The model under review builds one solid part; all positions refer to its coordinate system, in mm. Face numbers are marked on the shaded views. A direction names the side the tool comes from. Coordinates: 2 decimals unless noted, no trailing zeros. Loops run counter-clockwise (first coordinate to the right, second up) from the corner with the lowest first, then second, coordinate; pieces in that order, holes last. Notation, with made-up numbers: (6.25, -8.75) - (20.25, -8.75) arc R19 ccw to (20.25, -4.75) - close; hole circle Ø4 at (62, 21). An arc over 180 degrees is marked (long way). Use a Markdown table: item, result. Add a question column.
1) Clearance check with flat-ended pins moving along their axes: pin 1 (6 mm diameter, centred on y = -3.5, z = -8.5, fed in from +X); pin 2 (1.5 mm diameter, centred on y = 1.5, z = 15, fed in from -X); pin 3 (3 mm diameter, centred on x = -16.5, y = 6, fed in from +Z). State where each tip first meets the part, or that it passes through.
2) To check wall thickness, follow L1, parallel to Y at x = -23.9, z = 10.35; L2, parallel to Y at x = 23, z = 9; L3, parallel to Z at x = 23.5, y = 2. State the ranges of each line that lie inside material, in increasing order. Write a range as [from, to].
3) Add section B-B, the plane y = 5.1. Give the boundary of the cut face in (x, z).
4) Add section C-C, the plane x = 8. Give the boundary of the cut face in (y, z), and give its area (3 significant figures).
5) For the marked faces 1, 2, 3 and 4, list the 3-axis set-ups (+Z, -Z, +X, -X, +Y, -Y) from which the entire face can be reached by the end or side of a thin tool; tool diameter is ignored.
6) Add section A-A, the plane x = -23.9. Give the boundary of the cut face in (y, z).
7) Add section D-D, the plane z = 10.5. Give the boundary of the cut face in (x, y).
Autodesk Inventor part; units mm, degrees
ref_plane "YZ Plane" through (0, 0, 0) normal (1, 0, 0) x (0, 1, 0)
ref_plane "XZ Plane" through (0, 0, 0) normal (0, 1, 0) x (-1, 0, 0)
ref_plane "XY Plane" through (0, 0, 0) normal (0, 0, 1) x (1, 0, 0)
sketch "草圖1" plane through (0, 0, 0) normal (0, 1, 0) x (-1, 0, 0)
  line L0 (20, -18.25) -> (-20, -18.25)
  line L1 (-20, -18.25) -> (-20, 18.25)
  line L2 (-20, 18.25) -> (20, 18.25)
  line L3 (20, 18.25) -> (20, -18.25)
  line L4 (20, -18.25) -> (-20, 18.25) construction
  line L5 (-20, -18.25) -> (20, 18.25) construction
  line L6 (26.4, 11.25) -> (-26.4, 11.25)
  line L7 (-26.4, 11.25) -> (-26.4, 8.25)
  line L8 (-26.4, 8.25) -> (26.4, 8.25)
  line L9 (26.4, 8.25) -> (26.4, 11.25)
  point P0 (0, 0)
  point P1 (0, 11.25)
  point P2 (0, 18.25)
  dimension "d0" = 40
  dimension "d1" = 36.5
  dimension "d2" = 3
  dimension "d4" = 52.8
  dimension "d5" = 26.5
extrude "擠出1" add sketch "草圖1" along normal mid plane 20
sketch "草圖2" plane through (20, -10, 11.25) normal (0, 0, 1) x (1, 0, 0)
  line L0 (-40, 0) -> (-40, 20) construction
  line L1 (0, 20) -> (-40, 20) construction
  line L2 (0, 20) -> (0, 0) construction
  line L3 (-40, 0) -> (0, 0) construction
  line L4 (-43.9, 4.9) -> (3.9, 4.9) construction
  line L5 (3.9, 4.9) -> (3.9, 15.1) construction
  line L6 (3.9, 15.1) -> (-43.9, 15.1) construction
  line L7 (-43.9, 15.1) -> (-43.9, 4.9) construction
  line L8 (-43.9, 4.9) -> (3.9, 15.1) construction
  line L9 (3.9, 4.9) -> (-43.9, 15.1) construction
  point P0 (-20, 10)
  dimension "d8" = 47.8
  dimension "d9" = 10.2
hole "孔1" at (23.9, 5.1, 11.25) at (23.9, -5.1, 11.25) at (-23.9, -5.1, 11.25) at (-23.9, 5.1, 11.25) direction (0, 0, -1) diameter 5 depth 8 tip angle 118
sketch "草圖3" plane through (20, -10, 11.25) normal (0, 0, 1) x (1, 0, 0)
  circle A0 centre (3.9, 15.1) radius 2.5 construction
  line L0 (3.9, 16.6) -> (13.7017, 16.6)
  line L1 (13.7017, 16.6) -> (13.7017, 13.6)
  line L2 (13.7017, 13.6) -> (3.9, 13.6)
  line L3 (3.9, 13.6) -> (3.9, 16.6)
  point P0 (-20, 10)
  point P1 (6.4, 15.1)
  dimension "d17" = 3
extrude "擠出2" cut sketch "草圖3" against normal blind 20
mirror "鏡射1" about plane through (0, 0, 0) normal (0, 1, 0) of "擠出2"
mirror "鏡射2" about plane through (0, 0, 0) normal (1, 0, 0) of "擠出2", "鏡射1"
sketch "草圖4" plane through (-20, 10, 18.25) normal (0, 0, 1) x (1, 0, 0)
  circle A0 centre (28, -10) radius 2.5
  line L0 (40, 0) -> (40, -20) construction
  line L1 (0, 0) -> (0, -20)
  point P0 (20, -10)
  dimension "d20" = 5
  dimension "d25" = 12
extrude "擠出3" add sketch "草圖4" along normal blind 10
properties part number "馬達"
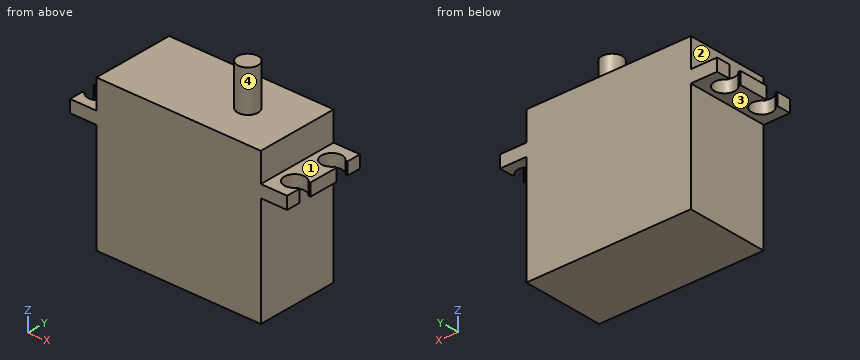
From the geometry:
| question | item | result |
|---|---|---|
| 1 | pin 1 | stops at x = 20 |
| 1 | pin 2 | stops at x = -20 |
| 1 | pin 3 | stops at z = 18.25 |
| 2 | L1 | y = [-10, -7.6], [-2.6, 2.6], [7.6, 10] |
| 2 | L2 | y = [-10, -7.43], [-2.77, 2.77], [7.43, 10] |
| 2 | L3 | z = [8.25, 11.25] |
| 3 | outline | (-21.4, 8.25) - (-20, 8.25) - (-20, -18.25) - (20, -18.25) - (20, 8.25) - (21.4, 8.25) - (21.4, 11.25) - (20, 11.25) - (20, 18.25) - (-20, 18.25) - (-20, 11.25) - (-21.4, 11.25) - close |
| 4 | outline | (-10, -18.25) - (10, -18.25) - (10, 18.25) - (2.5, 18.25) - (2.5, 28.25) - (-2.5, 28.25) - (-2.5, 18.25) - (-10, 18.25) - close |
| 4 | area | 780 mm^2 |
| 5 | face 1 | +Z, +X, +Y, -Y |
| 5 | face 2 | +Z, -X, +Y, -Y |
| 5 | face 3 | -Z, -X, +Y, -Y |
| 5 | face 4 | +Z |
| 6 | outline | (-10, 8.25) - (-7.6, 8.25) - (-7.6, 11.25) - (-10, 11.25) - close; (-2.6, 8.25) - (2.6, 8.25) - (2.6, 11.25) - (-2.6, 11.25) - close; (7.6, 8.25) - (10, 8.25) - (10, 11.25) - (7.6, 11.25) - close |
| 7 | outline | (-26.4, -10) - (26.4, -10) - (26.4, -6.6) - (25.9, -6.6) arc R2.5 cw (long way) to (25.9, -3.6) - (26.4, -3.6) - (26.4, 3.6) - (25.9, 3.6) arc R2.5 cw (long way) to (25.9, 6.6) - (26.4, 6.6) - (26.4, 10) - (-26.4, 10) - (-26.4, 6.6) - (-25.9, 6.6) arc R2.5 cw (long way) to (-25.9, 3.6) - (-26.4, 3.6) - (-26.4, -3.6) - (-25.9, -3.6) arc R2.5 cw (long way) to (-25.9, -6.6) - (-26.4, -6.6) - close |
